from build123d import *

# Parameters (mm, degrees)
SKETCH1_R           = 6.5
SKETCH1_R_2         = 5.5
SKETCH1_R_3         = 2.7
BOSS_EXTRUDE1_DEPTH = 3
BOSS_EXTRUDE2_START = -2
SKETCH1_3_R         = 6.5
SKETCH1_3_R_2       = 5.5
BOSS_EXTRUDE2_DEPTH = 2
CUT_EXTRUDE1_DEPTH  = 2
CIRPATTERN1_COUNT   = 8
FILLET2_R           = 0.4
CHAMFER1_SIZE       = 0.4


with BuildPart() as part:
    # Sketch1 → Boss-Extrude1 (new body)
    # profile 1 of 2: a face of its own
    with BuildSketch(Plane(origin=(0, 0, 0), x_dir=(1, 0, 0), z_dir=(0, 1, 0))):
        with Locations(Location((0, 0, 0), (0, 0, 270))):
            Circle(SKETCH1_R)
        Circle(SKETCH1_R_2, mode=Mode.SUBTRACT)
    # profile 2 of 2: a face of its own
    with BuildSketch(Plane(origin=(0, 0, 0), x_dir=(1, 0, 0), z_dir=(0, 1, 0))):
        Circle(SKETCH1_R_2)
        with Locations(Location((0, 0, 0), (0, 0, 270))):
            Circle(SKETCH1_R_3, mode=Mode.SUBTRACT)
    extrude(amount=BOSS_EXTRUDE1_DEPTH)

    # Sketch1_3 → Boss-Extrude2 (add)
    with BuildSketch(Plane(origin=(0, 0, 0), x_dir=(1, 0, 0), z_dir=(0, 1, 0)).offset(BOSS_EXTRUDE2_START)):
        with Locations(Location((0, 0, 0), (0, 0, 270))):
            Circle(SKETCH1_3_R)
        with Locations(Location((0, 0, 0), (0, 0, 270))):
            Circle(SKETCH1_3_R_2, mode=Mode.SUBTRACT)
    extrude(amount=BOSS_EXTRUDE2_DEPTH)

    # Sketch2 → Cut-Extrude1 (cut)
    with BuildSketch(Plane(origin=(0, -2, 0), x_dir=(-1, 0, 0), z_dir=(0, -1, 0))):
        Polygon((0, 0), (3.374998796, -5.555122242), (3.374998796, -6.374424951), (1.271497758, -6.374424951), align=None)
    cut_extrude1 = extrude(amount=-CUT_EXTRUDE1_DEPTH, mode=Mode.SUBTRACT)

    # CirPattern1: Cut-Extrude1 ×8 about axis
    cirpattern1_axis = Axis((0, 0, 0), (0, 1, 0))
    for i in range(1, CIRPATTERN1_COUNT):
        add(cut_extrude1.rotate(cirpattern1_axis, i * 360 / CIRPATTERN1_COUNT), mode=Mode.SUBTRACT)

    # Fillet2
    fillet2_edges = [part.edges().sort_by_distance(p)[0] for p in [
        (1.075882719, -1, -5.393744189),
        (1.271497758, -1, -6.374424951),
        (2.855768212, -1, -4.700488051),
        (3.374998796, -1, -5.555122242),
        (-3.053189126, -1, -4.574717058),
        (-3.608314421, -1, -5.406483796),
        (-1.304413907, -1, -5.343080044),
        (-1.541580072, -1, -6.314549143),
        (-5.393744189, -1, -1.075882719),
        (-6.374424951, -1, -1.271497758),
        (-4.700488051, -1, -2.855768212),
        (-5.555122242, -1, -3.374998796),
        (-4.574717058, -1, 3.053189126),
        (-5.406483796, -1, 3.608314421),
        (-5.343080044, -1, 1.304413907),
        (-6.314549143, -1, 1.541580072),
        (-1.075882719, -1, 5.393744189),
        (-1.271497758, -1, 6.374424951),
        (-2.855768212, -1, 4.700488051),
        (-3.374998796, -1, 5.555122242),
        (3.053189126, -1, 4.574717058),
        (3.608314421, -1, 5.406483796),
        (1.304413907, -1, 5.343080044),
        (1.541580072, -1, 6.314549143),
        (5.393744189, -1, 1.075882719),
        (6.374424951, -1, 1.271497758),
        (4.700488051, -1, 2.855768212),
        (5.555122242, -1, 3.374998796),
        (4.574717058, -1, -3.053189126),
        (5.406483796, -1, -3.608314421),
        (5.343080044, -1, -1.304413907),
        (6.314549143, -1, -1.541580072),
    ]]
    fillet(fillet2_edges, radius=FILLET2_R)

    # Chamfer1
    chamfer1_edges = [part.edges().sort_by_distance(p)[0] for p in [
        (0, 3, -6.5),
        (0, 3, -2.7),
    ]]
    chamfer(chamfer1_edges, length=CHAMFER1_SIZE)


solid = part.part
CAD build for the part. Positions are in the model's coordinates, mm. A direction names the side the tool comes from. Give positions to 0.01 mm unless a question says otherwise; leave off trailing zeros. Write each loop counter-clockwise with the first axis right and the second up, starting at its lowest first coordinate (ties: lowest second). Pieces come first, ordered by that corner, then holes. Notation, with made-up numbers: (65, 47.5) -> (77, 47.5) arc R23 cw to (77, 80.5) -> close; hole circle Ø7 at (-29.5, -30). An arc over 180 degrees is marked (long way). Return JSON: item names as keys, results as strings.
Item 1: Band-saw the part on C-C (y = -1.45). Give the number of separate pieces and of enclosed holes in the cut face, then the cut area to 3 significant figures.
Answer below:
{"separate pieces": "8", "enclosed holes": "0", "area": "19.8 mm2"}
Item 2: Drop flat-ended pins along their axis: pin 1 (3 mm diameter, centred on x = 2, y = 0, fed in from +Z); pin 2 (1 mm diameter, centred on y = 2.5, z = 4, fed in from +X). Give the stop position or say it passes through.
Answer below:
{"pin 1": "stops at z = 6.48", "pin 2": "stops at x = 5.48"}
Item 3: Band-saw the part on B-B (y = 1.9). List the corners of the cut face in (x, z), then the cut area to 3 significant figures.
Answer below:
{"outline": "circle Ø13 at (0, 0); hole circle Ø5.4 at (0, 0)", "area": "110 mm2"}
Item 4: Drill centre lines: probe 1 along X at (y, z) = (2, 0); probe 2 along Y at (x, z) = (3.75, 2.5); probe 3 along X at (y, z) = (-1.35, -4.5). Where is each one in solid material? Low to high.
Answer below:
{"probe 1": "x = -6.5 to -2.7, 2.7 to 6.5", "probe 2": "y = 0 to 3", "probe 3": "x = -4.69 to -3.24, 3.16 to 4.69"}
Item 5: Band-saw the part on A-A (z = 0). List the corners of the cut face in (x, y).
Answer below:
{"outline": "(-6.5, -2) -> (-5.5, -2) -> (-5.5, 0) -> (-2.7, 0) -> (-2.7, 2.6) -> (-3.1, 3) -> (-6.1, 3) -> (-6.5, 2.6) -> close; (2.7, 0) -> (5.5, 0) -> (5.5, -2) -> (6.5, -2) -> (6.5, 2.6) -> (6.1, 3) -> (3.1, 3) -> (2.7, 2.6) -> close"}
Item 6: Tool access for faces 1 (the cylindrical face through (-3.963, -1.014, -3.814)), 2 (the flat face through (-4, -2, -4)): list every direction of +Z, -Z, +X, -X, +Y, -Y with a clear straight run to the whole face (end or side of a thin tool).
Answer below:
{"face 1": "-Y", "face 2": "+Z, -Z, +X, -X, -Y"}
Item 7: Two-plate mould, pull along X, no slides. Class faces 3 (the cylindrical face through (3.963, -1.014, 3.814)), 4 (the flat face through (3, 3, 3)): +X half, -X half, draft (parallel to the pull), parting line (faces both ways), or undercut.
Answer below:
{"face 3": "undercut", "face 4": "draft"}
